For this review, use the dimensioned drawing (mm, ordinates from the lowest corner) and the shaded views. A direction names the side the tool comes from. Coordinates: 2 decimals unless noted, no trailing zeros. Loops run counter-clockwise (first coordinate to the right, second up) from the corner with the lowest first, then second, coordinate; pieces in that order, holes last. Notation, with made-up numbers: (30, -35.75) - (57, -35.75) arc R25 ccw to (57, -23.75) - close; hole circle Ø11 at (45, 9). An arc over 180 degrees is marked (long way). Answer in a Markdown table with one row per item. Add a question column.
(1) The part is to be moulded in two halves that separate along X. For the marked faces 1, 2, 3 and 4, say which applies: released by +X, released by -X, zero draft, split by the parting line, or undercut.
(2) For the marked faces 5, 6, 7, 8 and 9, list the 3-axis set-ups (+Z, -Z, +X, -X, +Y, -Y) from which the entire face can be reached by the end or side of a thin tool; tool diameter is ignored.
(3) We need section D-D, the plane x = 17.75. Write out the cut boundary in (y, z), plus the area to 3 significant figures.
(4) Clearance check with flat-ended pins moving along their axes: pin 1 (1.9 mm diameter, centred on x = 9, y = 9.5, fed in from +Z); pin 2 (3 mm diameter, centred on y = 9.5, z = 5.5, fed in from -X); pin 3 (3 mm diameter, centred on y = 5.5, z = 23.5, fed in from +X). State where each tip first meets the part, or that it passes through.
(5) We need section A-A, the plane x = 10. Write out the cut boundary in (y, z).
(6) We need section C-C, the plane z = 3.5. Write out the cut boundary in (x, y), plus the area to 3 significant figures.
(7) To check wall thickness, follow L1, parallel to Y at x = 10, z = 30; L2, parallel to Z at x = 11.25, y = 16.25; L3, parallel to Z at x = 11, y = 1. State the ranges of each line that lie inside material, in increasing order. Write a range as [from, to].
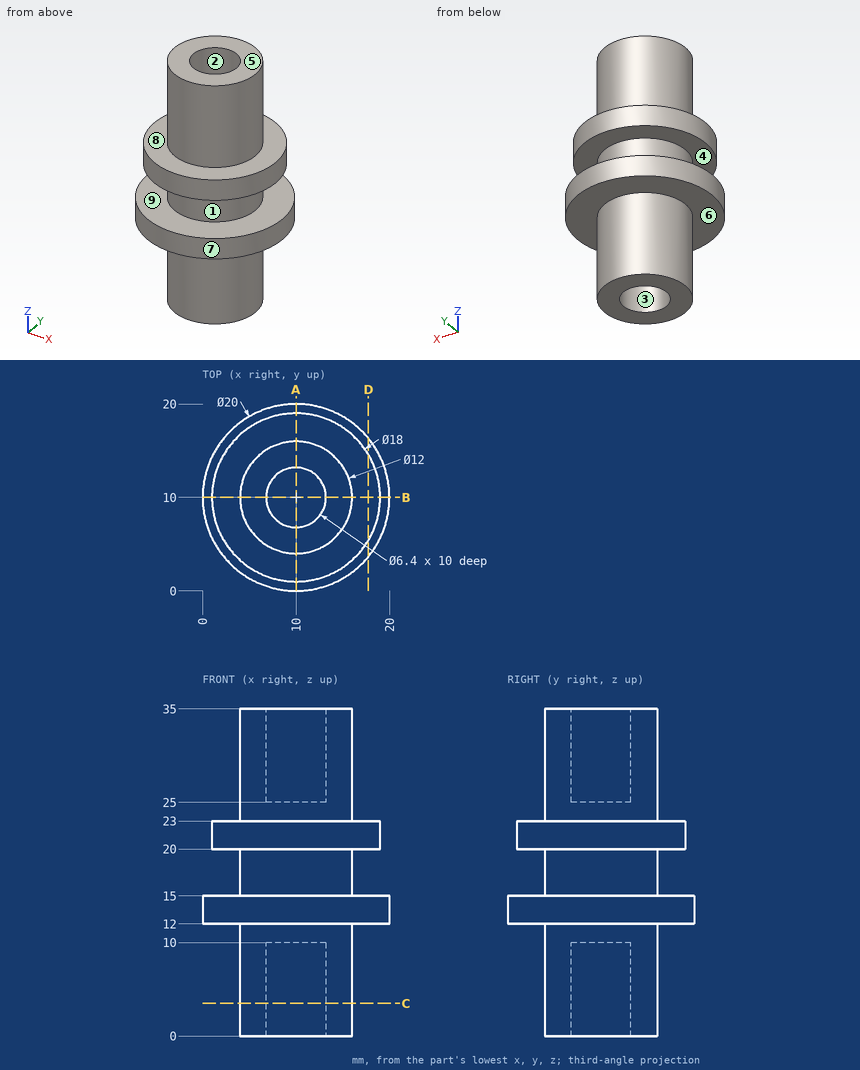
Responses:
| question | item | result |
|---|---|---|
| 1 | face 1 | split by the parting line |
| 1 | face 2 | undercut |
| 1 | face 3 | undercut |
| 1 | face 4 | zero draft |
| 2 | face 5 | +Z, +X, -X, +Y, -Y |
| 2 | face 6 | -Z |
| 2 | face 7 | +Z, -Z |
| 2 | face 8 | +Z |
| 2 | face 9 | none |
| 3 | outline | (3.68, 12) - (16.32, 12) - (16.32, 15) - (3.68, 15) - close; (5.42, 20) - (14.58, 20) - (14.58, 23) - (5.42, 23) - close |
| 3 | area | 65.4 mm2 |
| 4 | pin 1 | stops at z = 25 |
| 4 | pin 2 | stops at x = 4 |
| 4 | pin 3 | stops at x = 18.45 |
| 5 | outline | (0, 12) - (4, 12) - (4, 0) - (6.8, 0) - (6.8, 10) - (13.2, 10) - (13.2, 0) - (16, 0) - (16, 12) - (20, 12) - (20, 15) - (16, 15) - (16, 20) - (19, 20) - (19, 23) - (16, 23) - (16, 35) - (13.2, 35) - (13.2, 25) - (6.8, 25) - (6.8, 35) - (4, 35) - (4, 23) - (1, 23) - (1, 20) - (4, 20) - (4, 15) - (0, 15) - close |
| 6 | outline | circle Ø12 at (10, 10); hole circle Ø6.4 at (10, 10) |
| 6 | area | 80.9 mm2 |
| 7 | L1 | y = [4, 6.8], [13.2, 16] |
| 7 | L2 | z = [12, 15], [20, 23] |
| 7 | L3 | z = [12, 15] |
